from build123d import *

# Parameters (mm, degrees)
SKETCH1_W           = 200
SKETCH1_H           = 190
BOSS_EXTRUDE1_DEPTH = 4
BOSS_EXTRUDE2_DEPTH = 10
SKETCH4_R           = 50
CUT_EXTRUDE1_DEPTH  = 10
SKETCH9_W           = 200
SKETCH9_H           = 4
CUT_EXTRUDE6_DEPTH  = 12
SKETCH12_R          = 57.5
CUT_EXTRUDE7_DEPTH  = 2
SKETCH10_R          = 3
CUT_EXTRUDE8_DEPTH  = 10
CUT_EXTRUDE9_DEPTH  = 10


with BuildPart() as part:
    # Sketch1 → Boss-Extrude1 (new body)
    with BuildSketch(Plane(origin=(0, 0, 0), x_dir=(1, 0, 0), z_dir=(0, 1, 0))):
        with Locations((100, 95)):
            Rectangle(SKETCH1_W, SKETCH1_H)
    extrude(amount=BOSS_EXTRUDE1_DEPTH)

    # Sketch3 → Boss-Extrude2 (add)
    with BuildSketch(Plane(origin=(0, 4, 0), x_dir=(1, 0, 0), z_dir=(0, 1, 0))):
        with BuildLine():
            Line((30, 14.5), (18.788441151, 14.5))
            ThreePointArc((18.788441151, 14.5), (15.870102337, 16.769618143), (14.5, 20.203375202))
            Line((14.5, 20.203375202), (14.5, 30))
            ThreePointArc((14.5, 30), (10, 34.5), (5.5, 30))
            Line((5.5, 30), (5.5, 20.135411686))
            ThreePointArc((5.5, 20.135411686), (5.499816866, 19.870814738), (5.515185448, 19.60666443))
            ThreePointArc((5.515185448, 19.60666443), (8.973335462, 10.97845936), (16.633299171, 5.712561506))
            ThreePointArc((16.633299171, 5.712561506), (17.308434105, 5.553457904), (18, 5.5))
            Line((18, 5.5), (30, 5.5))
            ThreePointArc((30, 5.5), (34.5, 10), (30, 14.5))
        make_face()
        with BuildLine():
            Line((14.5, 190), (5.5, 190))
            Line((5.5, 190), (5.5, 155))
            ThreePointArc((5.5, 155), (10, 150.5), (14.5, 155))
            Line((14.5, 155), (14.5, 190))
        make_face()
        with BuildLine():
            Line((194.5, 155), (194.5, 190))
            Line((194.5, 190), (185.5, 190))
            Line((185.5, 190), (185.5, 155))
            ThreePointArc((185.5, 155), (190, 150.5), (194.5, 155))
        make_face()
        with BuildLine():
            Line((86.835483589, 190), (77.835483589, 190))
            Line((77.835483589, 190), (77.835483589, 175))
            ThreePointArc((77.835483589, 175), (82.335483589, 170.5), (86.835483589, 175))
            Line((86.835483589, 175), (86.835483589, 190))
        make_face()
        with BuildLine():
            Line((122.164516411, 175), (122.164516411, 190))
            Line((122.164516411, 190), (113.164516411, 190))
            Line((113.164516411, 190), (113.164516411, 175))
            ThreePointArc((113.164516411, 175), (117.664516411, 170.5), (122.164516411, 175))
        make_face()
        with BuildLine():
            Line((104.5, 190), (95.5, 190))
            Line((95.5, 190), (95.5, 170))
            ThreePointArc((95.5, 170), (100, 165.5), (104.5, 170))
            Line((104.5, 170), (104.5, 190))
        make_face()
        with BuildLine():
            Line((5.5, 90), (5.5, 50))
            ThreePointArc((5.5, 50), (10, 45.5), (14.5, 50))
            Line((14.5, 50), (14.5, 90))
            ThreePointArc((14.5, 90), (10, 94.5), (5.5, 90))
        make_face()
        with BuildLine():
            Line((70, 14.5), (50, 14.5))
            ThreePointArc((50, 14.5), (45.5, 10), (50, 5.5))
            Line((50, 5.5), (70, 5.5))
            ThreePointArc((70, 5.5), (74.5, 10), (70, 14.5))
        make_face()
        with BuildLine():
            ThreePointArc((185.5, 50), (190, 45.5), (194.5, 50))
            Line((194.5, 50), (194.5, 90))
            ThreePointArc((194.5, 90), (190, 94.5), (185.5, 90))
            Line((185.5, 90), (185.5, 50))
        make_face()
        with BuildLine():
            ThreePointArc((185.5, 20.203375202), (184.129897663, 16.769618143), (181.211558849, 14.5))
            Line((181.211558849, 14.5), (170, 14.5))
            ThreePointArc((170, 14.5), (165.5, 10), (170, 5.5))
            Line((170, 5.5), (182, 5.5))
            ThreePointArc((182, 5.5), (182.691565895, 5.553457904), (183.366700829, 5.712561506))
            ThreePointArc((183.366700829, 5.712561506), (191.026664538, 10.97845936), (194.484814552, 19.60666443))
            ThreePointArc((194.484814552, 19.60666443), (194.500183134, 19.870814738), (194.5, 20.135411686))
            Line((194.5, 20.135411686), (194.5, 30))
            ThreePointArc((194.5, 30), (190, 34.5), (185.5, 30))
            Line((185.5, 30), (185.5, 20.203375202))
        make_face()
        with BuildLine():
            ThreePointArc((150, 5.5), (154.5, 10), (150, 14.5))
            Line((150, 14.5), (130, 14.5))
            ThreePointArc((130, 14.5), (125.5, 10), (130, 5.5))
            Line((130, 5.5), (150, 5.5))
        make_face()
        with BuildLine():
            ThreePointArc((160.489637275, 46.636658066), (160.863341934, 52.989637275), (154.510362725, 53.363341934))
            Line((154.510362725, 53.363341934), (132.010362725, 33.363341934))
            ThreePointArc((132.010362725, 33.363341934), (131.636658066, 27.010362725), (137.989637275, 26.636658066))
            Line((137.989637275, 26.636658066), (160.489637275, 46.636658066))
        make_face()
        with BuildLine():
            Line((132.010362725, 156.636658066), (154.510362725, 136.636658066))
            ThreePointArc((154.510362725, 136.636658066), (160.863341934, 137.010362725), (160.489637275, 143.363341934))
            Line((160.489637275, 143.363341934), (137.989637275, 163.363341934))
            ThreePointArc((137.989637275, 163.363341934), (131.636658066, 162.989637275), (132.010362725, 156.636658066))
        make_face()
        with BuildLine():
            Line((5.5, 135), (5.5, 120))
            ThreePointArc((5.5, 120), (10, 115.5), (14.5, 120))
            Line((14.5, 120), (14.5, 135))
            ThreePointArc((14.5, 135), (10, 139.5), (5.5, 135))
        make_face()
        with BuildLine():
            ThreePointArc((39.510362725, 143.363341934), (39.136658066, 137.010362725), (45.489637275, 136.636658066))
            Line((45.489637275, 136.636658066), (67.989637275, 156.636658066))
            ThreePointArc((67.989637275, 156.636658066), (68.363341934, 162.989637275), (62.010362725, 163.363341934))
            Line((62.010362725, 163.363341934), (39.510362725, 143.363341934))
        make_face()
        with BuildLine():
            Line((67.989637275, 33.363341934), (45.489637275, 53.363341934))
            ThreePointArc((45.489637275, 53.363341934), (39.136658066, 52.989637275), (39.510362725, 46.636658066))
            Line((39.510362725, 46.636658066), (62.010362725, 26.636658066))
            ThreePointArc((62.010362725, 26.636658066), (68.363341934, 27.010362725), (67.989637275, 33.363341934))
        make_face()
        with BuildLine():
            ThreePointArc((185.5, 120), (190, 115.5), (194.5, 120))
            Line((194.5, 120), (194.5, 135))
            ThreePointArc((194.5, 135), (190, 139.5), (185.5, 135))
            Line((185.5, 135), (185.5, 120))
        make_face()
    extrude(amount=BOSS_EXTRUDE2_DEPTH)

    # Sketch4 → Cut-Extrude1 (cut)
    with BuildSketch(Plane(origin=(0, 0, 0), x_dir=(1, 0, 0), z_dir=(0, 1, 0))):
        with Locations(Location((100, 95, 0), (0, 0, 90))):
            Circle(SKETCH4_R)
    extrude(amount=CUT_EXTRUDE1_DEPTH, mode=Mode.SUBTRACT)

    # Sketch9 → Cut-Extrude6 (cut)
    with BuildSketch(Plane.XZ):
        with Locations((100, -2)):
            Rectangle(SKETCH9_W, SKETCH9_H)
    extrude(amount=-CUT_EXTRUDE6_DEPTH, mode=Mode.SUBTRACT)

    # Sketch12 → Cut-Extrude7 (cut)
    with BuildSketch(Plane(origin=(0, 0, 0), x_dir=(-1, 0, 0), z_dir=(0, -1, 0))):
        with Locations(Location((-100, 95, 0), (0, 0, 90))):
            Circle(SKETCH12_R)
    extrude(amount=-CUT_EXTRUDE7_DEPTH, mode=Mode.SUBTRACT)

    # Sketch10 → Cut-Extrude8 (cut)
    with BuildSketch(Plane(origin=(0, 4, 0), x_dir=(1, 0, 0), z_dir=(0, 1, 0))):
        with Locations(Location((10, 105, 0), (0, 0, 270))):
            Circle(SKETCH10_R)
        with Locations(Location((100, 20, 0), (0, 0, 270))):
            Circle(SKETCH10_R)
        with Locations(Location((190, 105, 0), (0, 0, 90))):
            Circle(SKETCH10_R)
    extrude(amount=-CUT_EXTRUDE8_DEPTH, mode=Mode.SUBTRACT)

    # Sketch13 → Cut-Extrude9 (cut)
    with BuildSketch(Plane.XZ):
        with BuildLine():
            ThreePointArc((49.5, -147.5), (48.914213562, -146.085786438), (47.5, -145.5))
            Line((47.5, -145.5), (47.5, -147.5))
            Line((47.5, -147.5), (49.5, -147.5))
        make_face()
        with BuildLine():
            Line((47.5, -147.5), (47.5, -145.5))
            ThreePointArc((47.5, -145.5), (46.085786438, -148.914213562), (49.5, -147.5))
            Line((49.5, -147.5), (47.5, -147.5))
        make_face()
        with BuildLine():
            ThreePointArc((47.5, -44.5021719), (48.914213562, -43.916385462), (49.5, -42.5021719))
            Line((49.5, -42.5021719), (47.5, -42.5021719))
            Line((47.5, -42.5021719), (47.5, -44.5021719))
        make_face()
        with BuildLine():
            Line((47.5, -42.5021719), (49.5, -42.5021719))
            ThreePointArc((49.5, -42.5021719), (46.085786438, -41.087958338), (47.5, -44.5021719))
            Line((47.5, -44.5021719), (47.5, -42.5021719))
        make_face()
        with BuildLine():
            ThreePointArc((154.4978281, -42.5021719), (152.4978281, -40.5021719), (150.4978281, -42.5021719))
            Line((150.4978281, -42.5021719), (152.4978281, -42.5021719))
            Line((152.4978281, -42.5021719), (152.4978281, -44.5021719))
            ThreePointArc((152.4978281, -44.5021719), (153.912041662, -43.916385462), (154.4978281, -42.5021719))
        make_face()
        with BuildLine():
            Line((152.4978281, -42.5021719), (150.4978281, -42.5021719))
            ThreePointArc((150.4978281, -42.5021719), (151.083614538, -43.916385462), (152.4978281, -44.5021719))
            Line((152.4978281, -44.5021719), (152.4978281, -42.5021719))
        make_face()
        with BuildLine():
            ThreePointArc((154.4978281, -147.5), (153.912041662, -146.085786438), (152.4978281, -145.5))
            Line((152.4978281, -145.5), (152.4978281, -147.5))
            Line((152.4978281, -147.5), (150.4978281, -147.5))
            ThreePointArc((150.4978281, -147.5), (152.4978281, -149.5), (154.4978281, -147.5))
        make_face()
        with BuildLine():
            Line((152.4978281, -147.5), (152.4978281, -145.5))
            ThreePointArc((152.4978281, -145.5), (151.083614538, -146.085786438), (150.4978281, -147.5))
            Line((150.4978281, -147.5), (152.4978281, -147.5))
        make_face()
    extrude(amount=-CUT_EXTRUDE9_DEPTH, mode=Mode.SUBTRACT)


solid = part.part
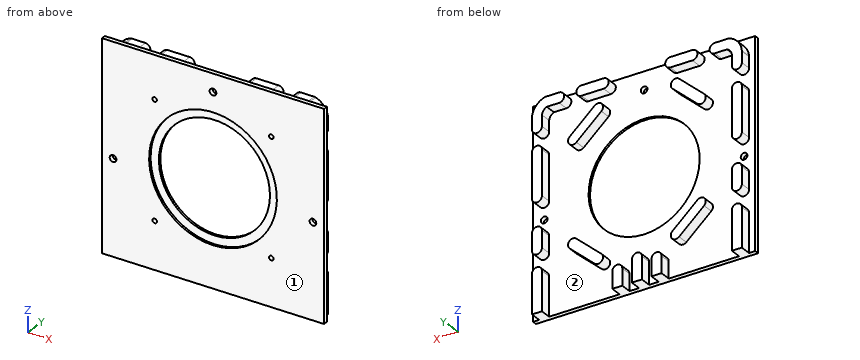
Could you check a few things on this model? Use its own coordinates, in mm. Face numbers are marked on the shaded views. Coordinates: 2 decimals unless noted, no trailing zeros. Order: outer loops, then holes, each group sorted by start corner. A loop starts at its lowest first (then second) coordinate and runs counter-clockwise, first axis right, second up. Notation, with made-up numbers: (-39.75, -7.5) - (11.25, -7.5) arc R11 ccw to (11.25, -0.5) - close; hole circle Ø9 at (43, 1). An arc over 180 degrees is marked (long way). Answer in a Markdown table with one row per item. Add a question column.
(1) If we section it at C-C, the plane z = -105: Please give me the cut outline in (x, y).
(2) Will these pins go through, and if not, where does the flat tip stop? pin 1 (3 mm diameter, centred on y = 8.5, z = -131, fed in from -X); pin 2 (5 mm diameter, centred on y = 10, z = -124, fed in from +X); pin 3 (3 mm diameter, centred on x = 25, y = 9, fed in from -Z).
(3) If we mould it in two halves opening along Z, with no side actions, what happens to the marked faces 1 and 2? For each: released by +Z, released by -Z, zero draft, split by the parting line, or undercut.
(4) If we section it at A-A, the plane y = 6.25: State how many separate pieces and enclosed holes the cut face has, then the cut area to 3 significant figures.
(5) If we section it at B-B, the plane x = 54: Please give me the cut outline in (y, z).
(6) I need wall thicknesses on L1, parallel to X at y = 9.25, z = -178.5; L2, parallel to Z at x = 47.5, y = 3; L3, parallel to X at y = 5.75, z = -62.5. Which ranges of each line are inside material? Lowest first, please.
(7) If we section it at D-D, the plane z = -60.5: Please give me the cut outline in (x, y).
Results are:
| question | item | result |
|---|---|---|
| 1 | outline | (0, 0) - (7, 0) - (7, 4) - (0, 4) - close; (13, 0) - (43.38, 0) - (43.38, 2) - (51.01, 2) - (51.01, 4) - (13, 4) - close; (148.99, 2) - (156.62, 2) - (156.62, 0) - (187, 0) - (187, 4) - (148.99, 4) - close; (193, 0) - (200, 0) - (200, 4) - (193, 4) - close |
| 2 | pin 1 | stops at x = 5.5 |
| 2 | pin 2 | stops at x = 194.5 |
| 2 | pin 3 | stops at z = -14.5 |
| 3 | face 1 | zero draft |
| 3 | face 2 | undercut |
| 4 | separate pieces | 17 |
| 4 | enclosed holes | 4 |
| 4 | area | 5,030 mm2 |
| 5 | outline | (0, -190) - (4, -190) - (4, -156.24) - (14, -156.24) - (14, -144.2) - (4, -144.2) - (4, -114.6) - (2, -114.6) - (2, -129.5) - (0, -129.5) - close; (0, -60.5) - (2, -60.5) - (2, -75.4) - (4, -75.4) - (4, -45.8) - (14, -45.8) - (14, -33.76) - (4, -33.76) - (4, -14.5) - (14, -14.5) - (14, -5.5) - (4, -5.5) - (4, -4) - (0, -4) - close |
| 6 | L1 | x = 5.5 to 14.5, 77.84 to 86.84, 95.5 to 104.5, 113.16 to 122.16, 185.5 to 194.5 |
| 6 | L2 | z = -190 to -149.5, -145.5 to -44.5, -40.5 to -4 |
| 6 | L3 | x = 5.5 to 14.5, 185.5 to 194.5 |
| 7 | outline | (0, 0) - (54, 0) - (54, 2) - (63.81, 2) - (63.81, 4) - (14.5, 4) - (14.5, 14) - (5.5, 14) - (5.5, 4) - (0, 4) - close; (136.19, 2) - (146, 2) - (146, 0) - (200, 0) - (200, 4) - (194.5, 4) - (194.5, 14) - (185.5, 14) - (185.5, 4) - (136.19, 4) - close |
